Read the model definition and answer for the solid it produces. Units are mm, in the model's axes. Face numbers are marked on the shaded views. Coordinates: 2 decimals unless noted, no trailing zeros. Order: outer loops, then holes, each group sorted by start corner. A loop starts at its lowest first (then second) coordinate and runs counter-clockwise, first axis right, second up. Notation, with made-up numbers: (-6.75, -17.75) -> (5.25, -17.75) arc R18 ccw to (5.25, 7.25) -> close; hole circle Ø2 at (-22, 30). An arc over 180 degrees is marked (long way). Use CSV: the item, a comma, the result in double quotes.
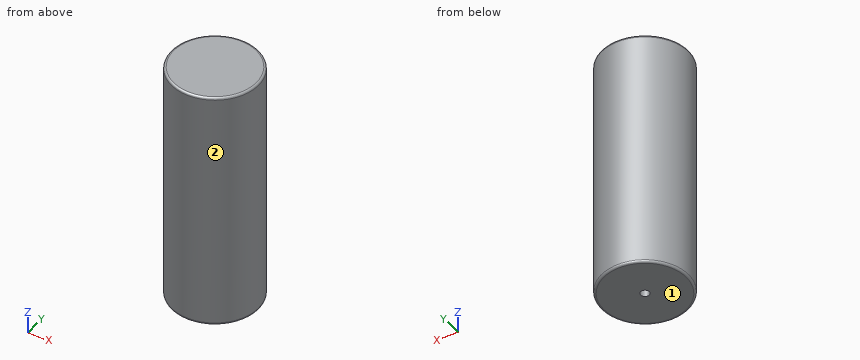
Autodesk Inventor part; units mm, degrees
ref_plane "YZ Plane" through (0, 0, 0) normal (1, 0, 0) x (0, 1, 0)
ref_plane "XZ Plane" through (0, 0, 0) normal (0, 1, 0) x (-1, 0, 0)
ref_plane "XY Plane" through (0, 0, 0) normal (0, 0, 1) x (1, 0, 0)
sketch "Sketch1" plane through (0, 0, 0) normal (0, 0, 1) x (1, 0, 0)
  circle A0 centre (0, 0) radius 31.75
  circle A1 centre (0, 0) radius 3.175
  dimension "d0" = 63.5
  dimension "d3" = 6.35
extrude "Extrusion1" add sketch "Sketch1" along normal blind 177.8 contours A0 | A1
extrude "Extrusion2" cut sketch "Sketch1" along normal blind 25.4 contours A1
thread "Thread1"
fillet "Fillet1" radius 1.5875 2 edges at (-31.75, 0, 177.8) (-31.75, 0, 0)
properties part number "Climber Extra Weight Cylinder" material "Aluminum 6061"
Item 1: The mould has two halves that part along X. Classify the marked faces 1 and 2: +X half, -X half, draft (parallel to the pull), parting line (faces both ways), or undercut.
Return value:
face 1,"draft"
face 2,"parting line"
Item 2: Find section A-A, the plane z = 124.5. Give the vertices of the cut face in (x, y), then the cut area to 3 significant figures.
Return value:
outline,"circle Ø63.5 at (0, 0)"
area,"3,170 mm^2"
Item 3: Straight lines are drawn through the part: line 1 along Y through (x, z) = (0, 13.75) (3 decimals); line 2 along Y through (x, z) = (-19.5, 123); line 3 along Y through (x, z) = (12, 14.5). For each, find the intervals that lie inside material, in ascending order.
Return value:
line 1,"y = -31.75 to -3.175, 3.175 to 31.75"
line 2,"y = -25.06 to 25.06"
line 3,"y = -29.39 to 29.39"
Item 4: Each of these flat-tipped pins is pushed along its axis until it touches: P1, Ø2, axis at x = 4.5, z = 131, coming from the +Y side; P2, Ø3, axis at x = -1, y = 0.5, coming from the -Z side; P3, Ø8, axis at y = 17, z = 76, coming from the -X side. Where does it stop, or does it pass through?
Return value:
P1,"stops at y = 31.56"
P2,"stops at z = 25.4"
P3,"stops at x = -28.97"
